```python
from build123d import *

# Parameters (mm, degrees)
F0_W      = 112.0901331306
F0_H      = 109.1817319393
F1_DEPTH  = 5.588
F2_W      = 101.775161922
F2_H      = 101.0821834207
F3_DEPTH  = 25.4
F4_W      = 4.89441026
F4_H      = 84.1260254383
F5_DEPTH  = 4.826
F7_W      = 106.8618372083
F7_H      = 106.4788401127
F8_DEPTH  = 2.794
F9_W      = 98.1444716454
F9_H      = 98.5935106874
F10_DEPTH = 25.4
F11_W     = 7.0638842881
F11_H     = 11.2456418574
F12_DEPTH = 1.778
F15_W     = 112.0901331306
F15_H     = 109.1817319393
F15_W_2   = 101.775161922
F15_H_2   = 101.0821834207
F16_DEPTH = 1.016


with BuildPart() as f1:
    # F0 (on Top) → F1 (new body)
    with BuildSketch(Plane.XY):
        Rectangle(F0_W, F0_H)
    extrude(amount=F1_DEPTH)

    # F2 (on face) → F3 (cut)
    with BuildSketch(Plane.XY.offset(5.588)):
        Rectangle(F2_W, F2_H)
    extrude(amount=-F3_DEPTH, mode=Mode.SUBTRACT)

    # F4 (on face) → F5 (join)
    with BuildSketch(Plane.YZ.offset(56.0450665653)):
        with Locations((2.44720513, -42.0630127192)):
            Rectangle(F4_W, F4_H)
    extrude(amount=-F5_DEPTH)

    # F6: F1 across plane


with BuildPart() as f1_1:
    add(f1.part)
    add(f1.part.mirror(Plane.YZ))

    # F7 (on face) → F8 (join)
    with BuildSketch(Plane(origin=(0, 0, -84.1260254383), x_dir=(1, 0, 0), z_dir=(0, 0, -1))):
        Rectangle(F7_W, F7_H)
    extrude(amount=F8_DEPTH)

    # F9 (on face) → F10 (cut)
    with BuildSketch(Plane(origin=(0, 0, -86.9200254383), x_dir=(1, 0, 0), z_dir=(0, 0, -1))):
        Rectangle(F9_W, F9_H)
    extrude(amount=-F10_DEPTH, mode=Mode.SUBTRACT)

    # F11 (on face) → F12 (join)
    with BuildSketch(Plane(origin=(0, 0, -86.9200254383), x_dir=(1, 0, 0), z_dir=(0, 0, -1))):
        Polygon((-53.4309186041, -38.0511134863), (-53.4309186041, -53.2394200563), (-42.0083515346, -53.2394200563), (-42.0083515346, -49.2967553437), (-49.0722358227, -49.2967553437), (-49.0722358227, -38.0511134863), align=None)
        with Locations((-45.5402936786, -43.673934415)):
            Rectangle(F11_W, F11_H)
    extrude(amount=F12_DEPTH)

    # F13: F1 across plane


with BuildPart() as f1_2:
    add(f1_1.part)
    add(f1_1.part.mirror(Plane.XZ))

    # F14: F1 across plane


with BuildPart() as f1_3:
    add(f1_2.part)
    add(f1_2.part.mirror(Plane.YZ))

    # F15 (on face) → F16 (join)
    with BuildSketch(Plane.XY.offset(5.588)):
        Rectangle(F15_W, F15_H)
        Rectangle(F15_W_2, F15_H_2, mode=Mode.SUBTRACT)
    extrude(amount=-F16_DEPTH)


solid = f1_3.part
```
CAD build for the part. Positions are in the model's coordinates, mm. A direction names the side the tool comes from. Coordinates: 2 decimals unless noted, no trailing zeros. Order: outer loops, then holes, each group sorted by start corner. A loop starts at its lowest first (then second) coordinate and runs counter-clockwise, first axis right, second up.
(1) Saw through at C-C, the plane y = 42.5. Write the cut outline in (x, z).
Solution:
outline: (-56.05, 0) - (-50.89, 0) - (-50.89, 5.59) - (-56.05, 5.59) - close; (-53.43, -88.7) - (-42.01, -88.7) - (-42.01, -86.92) - (-49.07, -86.92) - (-49.07, -84.13) - (-53.43, -84.13) - close; (42.01, -88.7) - (53.43, -88.7) - (53.43, -84.13) - (49.07, -84.13) - (49.07, -86.92) - (42.01, -86.92) - close; (50.89, 0) - (56.05, 0) - (56.05, 5.59) - (50.89, 5.59) - close
(2) Saw through at A-A, the plane y = 3. Write the cut outline in (x, z).
Solution:
outline: (-56.05, -84.13) - (-53.43, -84.13) - (-53.43, -86.92) - (-49.07, -86.92) - (-49.07, -84.13) - (-51.22, -84.13) - (-51.22, 0) - (-50.89, 0) - (-50.89, 5.59) - (-56.05, 5.59) - close; (49.07, -86.92) - (53.43, -86.92) - (53.43, -84.13) - (56.05, -84.13) - (56.05, 5.59) - (50.89, 5.59) - (50.89, 0) - (51.22, 0) - (51.22, -84.13) - (49.07, -84.13) - close
(3) Saw through at B-B, the plane x = 45. Write the cut outline in (y, z), and give its area (3 significant figures).
Solution:
outline: (-54.59, 0) - (-50.54, 0) - (-50.54, 5.59) - (-54.59, 5.59) - close; (-53.24, -88.7) - (-38.05, -88.7) - (-38.05, -86.92) - (-49.3, -86.92) - (-49.3, -84.13) - (-53.24, -84.13) - close; (38.05, -88.7) - (53.24, -88.7) - (53.24, -84.13) - (49.3, -84.13) - (49.3, -86.92) - (38.05, -86.92) - close; (50.54, 0) - (54.59, 0) - (54.59, 5.59) - (50.54, 5.59) - close
area: 121 mm2
(4) Mould opens along X. For faces 4 (the face through (-4, -52, 5.588)), 5 (the face through (56.045, 0, -26)), 6 (the face through (-1, -50.541, 3)) say: released by +X, released by -X, zero draft, split by the parting line, or undercut.
Solution:
face 4: zero draft
face 5: released by +X
face 6: undercut
(5) Which spindle directions (+Z, -Z, +X, -X, +Y, -Y) get a long thin tool onto all of the face, cutting with end or side? Do faces 1 (the face through (-1, 53.239, -86)), 2 (the face through (50.888, -1, 3)), 3 (the face through (-51, -1, -86.92)). Say none if no direction does.
Solution:
face 1: -Z, +X, -X, +Y
face 2: +Z
face 3: -Z, +X, -X
(6) Drill centre lines: L1, parallel to Y at x = -46, z = 0.5; L2, parallel to Z at x = -44.5, y = -39; L3, parallel to Z at x = 3.5, y = 50.5. Where is each one in solid material? Low to high.
Solution:
L1: y = -54.59 to -50.54, 50.54 to 54.59
L2: z = -88.7 to -86.92
L3: z = -86.92 to -84.13
(7) Pin check, flat tips, straight feed: pin 1 Ø4 at (x, z) = (53.5, -27.5) entering from -Y; pin 2 Ø0.9 at (x, z) = (-46.5, -88) entering from -Y; pin 3 Ø3.5 at (x, y) = (51.5, -5) entering from -Z; pin 4 Ø6 at (x, y) = (8.5, 43.5) entering from -Z. Stop position of each tip, or through.
Solution:
pin 1: stops at y = -4.89
pin 2: stops at y = -53.24
pin 3: stops at z = -86.92
pin 4: passes through
(8) Saw through at D-D, the plane z = -6.5. Write the cut outline in (x, y).
Solution:
outline: (-56.05, -4.89) - (-51.22, -4.89) - (-51.22, 4.89) - (-56.05, 4.89) - close; (51.22, -4.89) - (56.05, -4.89) - (56.05, 4.89) - (51.22, 4.89) - close
